```python
from build123d import *

# Parameters (mm, degrees)
BASE_FLANGE1_DEPTH   = 30
EDGE_FLANGE1_DEPTH   = 35
EDGE_FLANGE1_START   = 31.38558
EDGE_FLANGE1_2_DEPTH = 3.61442
EDGE_FLANGE1_3_DEPTH = 31.38558


# Read off the part's stored shape, not the designer's step: Edge-Flange1
# Sheet-metal steps are written as plain solids
with BuildPart() as part:
    # Sketch1 → Base-Flange1 (new body)
    with BuildSketch(Plane.XY):
        with BuildLine():
            Line((-30, 35), (-3.61442, 35))
            ThreePointArc((-3.61442, 35), (-1.058639108, 33.941360892), (0, 31.38558))
            Line((0, 31.38558), (0, 0))
            Line((0, 0), (-1.70942, 0))
            Line((-1.70942, 0), (-1.70942, 31.38558))
            ThreePointArc((-1.70942, 31.38558), (-2.267381582, 32.732618418), (-3.61442, 33.29058))
            Line((-3.61442, 33.29058), (-30, 33.29058))
            Line((-30, 33.29058), (-30, 35))
        make_face()
    extrude(amount=BASE_FLANGE1_DEPTH)

    # Edge-Flange1 outline → Edge-Flange1 (cut)
    with BuildSketch(Plane(origin=(0, 0, 0), x_dir=(1, 0, 0), z_dir=(0, 1, 0))):
        with BuildLine():
            Line((-3.61442, -30), (0, -30))
            Line((0, -30), (0, -26.38558))
            ThreePointArc((0, -26.38558), (-1.058639108, -28.941360892), (-3.61442, -30))
        make_face()
        with BuildLine():
            Line((-3.61442, -26.38558), (-3.61442, -28.29058))
            ThreePointArc((-3.61442, -28.29058), (-2.267381582, -27.732618418), (-1.70942, -26.38558))
            Line((-1.70942, -26.38558), (-3.61442, -26.38558))
        make_face()
    extrude(amount=EDGE_FLANGE1_DEPTH, mode=Mode.SUBTRACT)

    # Edge-Flange1 2 outline → Edge-Flange1 2 (cut)
    with BuildSketch(Plane(origin=(0, 0, 0), x_dir=(1, 0, 0), z_dir=(0, 1, 0)).offset(EDGE_FLANGE1_START)):
        with BuildLine():
            Line((-3.61442, -28.29058), (-3.61442, -30))
            ThreePointArc((-3.61442, -30), (-1.058639108, -28.941360892), (0, -26.38558))
            Line((0, -26.38558), (-1.70942, -26.38558))
            ThreePointArc((-1.70942, -26.38558), (-2.267381582, -27.732618418), (-3.61442, -28.29058))
        make_face()
    extrude(amount=EDGE_FLANGE1_2_DEPTH, mode=Mode.SUBTRACT)

    # Edge-Flange1 3 outline → Edge-Flange1 3 (add)
    with BuildSketch(Plane(origin=(0, 0, 0), x_dir=(1, 0, 0), z_dir=(0, 1, 0))):
        with BuildLine():
            Line((-20, -30), (-3.61442, -30))
            ThreePointArc((-3.61442, -30), (-2.624012381, -29.861658924), (-1.70942, -29.45722564))
            Line((-1.70942, -29.45722564), (-1.70942, -26.38558))
            ThreePointArc((-1.70942, -26.38558), (-2.267381582, -27.732618418), (-3.61442, -28.29058))
            Line((-3.61442, -28.29058), (-20, -28.29058))
            Line((-20, -28.29058), (-20, -30))
        make_face()
    extrude(amount=EDGE_FLANGE1_3_DEPTH)


solid = part.part
```
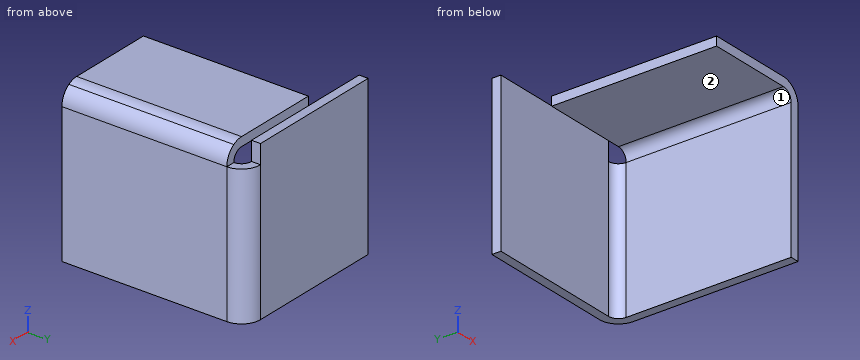
For this review, take the finished solid that the model builds, in its own axes (mm). Face numbers are marked on the shaded views. A direction names the side the tool comes from. Give positions to 0.01 mm unless a question says otherwise; leave off trailing zeros. Order: outer loops, then holes, each group sorted by start corner. A loop starts at its lowest first (then second) coordinate and runs counter-clockwise, first axis right, second up.
1) Insertion check: pin 1 (0.5 mm diameter, centred on y = 16.5, z = 29.5, fed in from -X); pin 2 (1.1 mm diameter, centred on x = -2, y = 32.5, fed in from +Z); pin 3 (10 mm diameter, centred on x = -7.5, z = 14, fed in from -Y). Each pin has a flat end and moves straight along its axis. Give the tip position at first contact, or say it passes through.
2) Wall thickness on line 1 (Z direction, x = -4, y = 27); line 2 (X direction, y = 17, z = 2); line 3 (Y direction, x = -18.75, z = 28.75): over which ranges is each line inside the solid? List them lowest first.
3) Take a section at A-A (x = -6). Give the boundary of the cut face in (y, z), then the cut area to 3 significant figures.
4) Take a section at D-D (z = 15.5). Give the boundary of the cut face in (x, y) (3 decimals).
5) Take a section at B-B (z = 27.25). Give the boundary of the cut face in (x, y), then the cut area to 3 significant figures.
6) For the marked faces 1 and 2, list the 3-axis set-ups (+Z, -Z, +X, -X, +Y, -Y) from which the entire face can be reached by the end or side of a thin tool; tool diameter is ignored.
7) Take a section at C-C (y = 6). Give the boundary of the cut face in (x, z) (3 decimals), then the cut area to 3 significant figures.
Derived:
1. pin 1: stops at x = -20
1. pin 2: stops at z = 26.39
1. pin 3: stops at y = 32.93
2. line 1: z = 28.29 to 30
2. line 2: x = -1.71 to 0
2. line 3: y = 0 to 31.39, 33.29 to 35
3. outline: (0, 28.29) - (31.39, 28.29) - (31.39, 30) - (0, 30) - close; (33.29, 0) - (35, 0) - (35, 30) - (33.29, 30) - close
3. area: 105 mm2
4. outline: (-30, 33.291) - (-3.614, 33.291) arc R1.905 cw to (-1.709, 31.386) - (-1.709, 0) - (0, 0) - (0, 31.386) arc R3.614 ccw to (-3.614, 35) - (-30, 35) - close
5. outline: (-30, 33.29) - (-3.61, 33.29) - (-3.61, 35) - (-30, 35) - close; (-1.92, 0) - (-0.1, 0) - (-0.1, 31.39) - (-1.92, 31.39) - close
5. area: 102 mm2
6. face 1: -Z, -X, +Y, -Y
6. face 2: -Z, -X, -Y
7. outline: (-20, 28.291) - (-3.614, 28.291) arc R1.905 cw to (-1.709, 26.386) - (-1.709, 0) - (0, 0) - (0, 26.386) arc R3.614 ccw to (-3.614, 30) - (-20, 30) - close
7. area: 80.5 mm2
